Verification items for the finished model (mm, model axes). A direction names the side the tool comes from. Give positions to 0.01 mm unless a question says otherwise; leave off trailing zeros. Write each loop counter-clockwise with the first axis right and the second up, starting at its lowest first coordinate (ties: lowest second). Pieces come first, ordered by that corner, then holes. Notation, with made-up numbers: M 25.25,47 L 52.25,47 A19 ccw 52.25,71 Z; hole C 44.5,2.5 d9. An arc over 180 degrees is marked long. Write item = value, one per line.
from build123d import *

# Parameters (mm, degrees)
F0_W     = 6.35
F0_H     = 6.35
F0_W_2   = 3.2385
F0_H_2   = 3.2385
F1_DEPTH = 31.75
F2_SIZE  = 1.27


with BuildPart() as f1:
    # F0 (on Front) → F1 (new body)
    with BuildSketch(Plane.XZ):
        Rectangle(F0_W, F0_H)
        Rectangle(F0_W_2, F0_H_2, mode=Mode.SUBTRACT)
    extrude(amount=F1_DEPTH)

    # F2
    f2_edges = [f1.edges().sort_by_distance(p)[0] for p in [
        (3.175, -15.875, 3.175),
        (3.175, -15.875, -3.175),
        (-3.175, -15.875, -3.175),
        (-3.175, -15.875, 3.175),
    ]]
    chamfer(f2_edges, length=F2_SIZE)


solid = f1.part
1) Cross-section at C-C on y = -28. Record the boundary of the cut face in (x, z) (3 decimals), plus the area to 3 significant figures.
From the geometry:
outline = M -3.175,-1.905 L -1.905,-3.175 L 1.905,-3.175 L 3.175,-1.905 L 3.175,1.905 L 1.905,3.175 L -1.905,3.175 L -3.175,1.905 Z; hole M -1.619,-1.619 L 1.619,-1.619 L 1.619,1.619 L -1.619,1.619 Z
area = 26.6 mm^2
2) Tool access check on faces 4 (the flat face through (0, -16, -3.175)), 5 (the flat face through (-1.619, -16, 0)). Record the directions out of +Z, -Z, +X, -X, +Y, -Y that give a thin tool (end or side, any length) a straight path to the whole face; none if there is none.
From the geometry:
face_4 = -Z, +X, -X, +Y, -Y
face_5 = +Y, -Y
3) Cross-section at D-D on x = -2.25. Record the boundary of the cut face in (y, z), plus the area to 3 significant figures.
From the geometry:
outline = M -31.75,-2.83 L 0,-2.83 L 0,2.83 L -31.75,2.83 Z
area = 180 mm^2
4) Cross-section at A-A on z = 1. Record the boundary of the cut face in (x, y) (3 decimals).
From the geometry:
outline = M -3.175,-31.75 L -1.619,-31.75 L -1.619,0 L -3.175,0 Z; M 1.619,-31.75 L 3.175,-31.75 L 3.175,0 L 1.619,0 Z
5) Cross-section at B-B on x = 0. Record the boundary of the cut face in (y, z) (3 decimals).
From the geometry:
outline = M -31.75,-3.175 L 0,-3.175 L 0,-1.619 L -31.75,-1.619 Z; M -31.75,1.619 L 0,1.619 L 0,3.175 L -31.75,3.175 Z
6) Draft check along Z on faces 1 (the flat face through (0, -16, -1.619)), 2 (the flat face through (-3.175, -16, 0)), 3 (the flat face through (-2.53, -15.65, -2.55)). Enter one of: +Z half, -Z half, draft (parallel to the pull), parting line (faces both ways), or undercut.
From the geometry:
face_1 = undercut
face_2 = draft
face_3 = -Z half
7) Material ranges on probe 1 along X at (y, z) = (-4, 1.25) (3 decimals); probe 2 along Z at (x, y) = (2.25, -6), recorded low to high. Write a range as from..to.
From the geometry:
probe_1 = -3.175..-1.619, 1.619..3.175
probe_2 = -2.83..2.83
